from build123d import *

# Parameters (mm, degrees)
SKETCH1_R               = 2.25
BOSS_EXTRUDE1_DEPTH     = 38
CUT_EXTRUDE1_DEPTH      = 75.121521841
CUT_EXTRUDE1_DEPTH_BACK = 75.121521841


with BuildPart() as part:
    # Sketch1 → Boss-Extrude1 (new body)
    with BuildSketch(Plane(origin=(0, 0, 0), x_dir=(1, 0, 0), z_dir=(0, 1, 0))):
        with BuildLine():
            Line((-35.75, -40), (35.75, -40))
            ThreePointArc((35.75, -40), (38.75520382, -38.75520382), (40, -35.75))
            Line((40, -35.75), (40, 35.75))
            ThreePointArc((40, 35.75), (38.75520382, 38.75520382), (35.75, 40))
            Line((35.75, 40), (-35.75, 40))
            ThreePointArc((-35.75, 40), (-38.75520382, 38.75520382), (-40, 35.75))
            Line((-40, 35.75), (-40, -35.75))
            ThreePointArc((-40, -35.75), (-38.75520382, -38.75520382), (-35.75, -40))
        make_face()
        with Locations(Location((35.75, 35.75, 0), (0, 0, 270))):
            Circle(SKETCH1_R, mode=Mode.SUBTRACT)
        with Locations(Location((35.75, -35.75, 0), (0, 0, 270))):
            Circle(SKETCH1_R, mode=Mode.SUBTRACT)
        with Locations(Location((-35.75, -35.75, 0), (0, 0, 270))):
            Circle(SKETCH1_R, mode=Mode.SUBTRACT)
        with Locations(Location((-35.75, 35.75, 0), (0, 0, 270))):
            Circle(SKETCH1_R, mode=Mode.SUBTRACT)
        with BuildLine():
            Line((22.009940936, 39.25), (-22.009940936, 39.25))
            ThreePointArc((-22.009940936, 39.25), (-31.819805153, 31.819805153), (-39.25, 22.009940936))
            Line((-39.25, 22.009940936), (-39.25, -22.009940936))
            ThreePointArc((-39.25, -22.009940936), (-31.819805153, -31.819805153), (-22.009940936, -39.25))
            Line((-22.009940936, -39.25), (22.009940936, -39.25))
            ThreePointArc((22.009940936, -39.25), (31.819805153, -31.819805153), (39.25, -22.009940936))
            Line((39.25, -22.009940936), (39.25, 22.009940936))
            ThreePointArc((39.25, 22.009940936), (31.819805153, 31.819805153), (22.009940936, 39.25))
        make_face(mode=Mode.SUBTRACT)
    extrude(amount=BOSS_EXTRUDE1_DEPTH)

    # Sketch2 → Revolve1 (revolve)
    with BuildSketch(Plane(origin=(0, 0, 0), x_dir=(0, 0, -1), z_dir=(1, 0, 0))):
        Polygon((45, 4), (39.25, 9.75), (39.25, 28.25), (45, 34), align=None)
    revolve(axis=Axis((0, 0, 0), (0, 1, 0)))

    # Sketch3 → Cut-Extrude1 (cut, two sides: drawn at the far end of the back side and taken through both)
    with BuildSketch(Plane(origin=(0, 0, 0), x_dir=(1, 0, 0), z_dir=(0, 1, 0)).offset(-CUT_EXTRUDE1_DEPTH_BACK)):
        with BuildLine():
            Line((-40, -35.75), (-40, 35.75))
            ThreePointArc((-40, 35.75), (-39.676488013, 37.376404588), (-38.75520382, 38.75520382))
            ThreePointArc((-38.75520382, 38.75520382), (-54.808134855, 0), (-38.75520382, -38.75520382))
            ThreePointArc((-38.75520382, -38.75520382), (-39.676488013, -37.376404588), (-40, -35.75))
        make_face()
        with BuildLine():
            ThreePointArc((-35.75, -40), (-37.376404588, -39.676488013), (-38.75520382, -38.75520382))
            ThreePointArc((-38.75520382, -38.75520382), (6e-09, -54.808134855), (38.755203828, -38.755203812))
            ThreePointArc((38.755203828, -38.755203812), (37.376404593, -39.676488011), (35.75, -40))
            Line((35.75, -40), (-35.75, -40))
        make_face()
        with BuildLine():
            ThreePointArc((54.808134855, 0), (50.636113998, 20.97416519), (38.755203786, 38.755203854))
            ThreePointArc((38.755203786, 38.755203854), (39.676488004, 37.376404609), (40, 35.75))
            Line((40, 35.75), (40, -35.75))
            ThreePointArc((40, -35.75), (39.676488015, -37.376404582), (38.755203828, -38.755203812))
            ThreePointArc((38.755203828, -38.755203812), (50.63611401, -20.974165163), (54.808134855, 0))
        make_face()
        with BuildLine():
            ThreePointArc((38.755203786, 38.755203854), (-2.4e-08, 54.808134855), (-38.75520382, 38.75520382))
            ThreePointArc((-38.75520382, 38.75520382), (-37.376404588, 39.676488013), (-35.75, 40))
            Line((-35.75, 40), (35.75, 40))
            ThreePointArc((35.75, 40), (37.376404566, 39.676488022), (38.755203786, 38.755203854))
        make_face()
    extrude(amount=CUT_EXTRUDE1_DEPTH + CUT_EXTRUDE1_DEPTH_BACK, mode=Mode.SUBTRACT)


solid = part.part
Check sheet for the modelled part. Datum: model origin and axes. Units: mm. A direction names the side the tool comes from. Round coordinates to 2 decimals unless told otherwise and drop trailing zeros. Loops run counter-clockwise (first coordinate to the right, second up) from the corner with the lowest first, then second, coordinate; pieces in that order, holes last. Notation, with made-up numbers: (-34, -36.5) -> (7, -36.5) arc R13 cw to (7, -18.5) -> close; hole circle Ø4 at (57, -25). An arc over 180 degrees is marked (long way). Put each result on its own line as item: value. Start each with the question number.
1. Section check B-B (y = 17). Enter the section's corners in (x, z).
2. Draft check along Z on faces 1 (the face through (1, 19, -40)), 2 (the face through (31.7, 1.97, 31.94)), 3 (the face through (-38.79, 18.73, 38.72)). Enter one of: +Z half, -Z half, draft (parallel to the pull), parting line (faces both ways), or undercut.
3. Section check A-A (y = 35). Enter the section's corners in (x, z).
4. Gauge pin test, flat ends, axial feed: pin 1 (2.5 mm diameter, centred on x = -35.75, z = 35.75, fed in from +Y); pin 2 (12 mm diameter, centred on x = -21.5, z = -31, fed in from -Y). Record the tip position at first contact, or that the pin passes through.
5. Scan lines: probe 1 along X at (y, z) = (29, 1); probe 2 along Z at (x, y) = (-35.5, 18.5). Record each from-to range of solid material in increasing order.
6. Access from +Z, -Z, +X, -X, +Y, -Y to the whole of each face (thin tool, end or side, straight path). Record for faces 4 (the face through (-1.73, 19.13, 39.21)), 5 (the face through (28.59, 29.89, 29.23)), 6 (the face through (-29.17, 8.19, 28.54)).
Findings:
1. outline: (-40, -35.75) arc R4.25 ccw to (-35.75, -40) -> (35.75, -40) arc R4.25 ccw to (40, -35.75) -> (40, 35.75) arc R4.25 ccw to (35.75, 40) -> (-35.75, 40) arc R4.25 ccw to (-40, 35.75) -> close; hole circle Ø78.5 at (0, 0); hole circle Ø4.5 at (-35.75, -35.75); hole circle Ø4.5 at (-35.75, 35.75); hole circle Ø4.5 at (35.75, -35.75); hole circle Ø4.5 at (35.75, 35.75)
2. face 1: -Z half
2. face 2: undercut
2. face 3: +Z half
3. outline: (-40, -35.75) arc R4.25 ccw to (-35.75, -40) -> (35.75, -40) arc R4.25 ccw to (40, -35.75) -> (40, 35.75) arc R4.25 ccw to (35.75, 40) -> (-35.75, 40) arc R4.25 ccw to (-40, 35.75) -> close; hole (-39.25, -22.01) arc R45 ccw to (-22.01, -39.25) -> (22.01, -39.25) arc R45 ccw to (39.25, -22.01) -> (39.25, 22.01) arc R45 ccw to (22.01, 39.25) -> (-22.01, 39.25) arc R45 ccw to (-39.25, 22.01) -> close; hole circle Ø4.5 at (-35.75, -35.75); hole circle Ø4.5 at (-35.75, 35.75); hole circle Ø4.5 at (35.75, -35.75); hole circle Ø4.5 at (35.75, 35.75)
4. pin 1: passes through
4. pin 2: stops at y = 5.27
5. probe 1: x = -40 to -39.25, 39.25 to 40
5. probe 2: z = -40 to -37.99, -33.51 to -16.74, 16.74 to 33.51, 37.99 to 40
6. face 4: +Y, -Y
6. face 5: +Y
6. face 6: -Y
